```python
from build123d import *

# Parameters (mm, degrees)
SKETCH1_R           = 1.5
BOSS_EXTRUDE1_DEPTH = 5
SKETCH2_W           = 3.5
SKETCH2_H           = 1.5
CUT_EXTRUDE1_DEPTH  = 32.689903755


with BuildPart() as part:
    # Sketch1 → Boss-Extrude1 (new body)
    with BuildSketch(Plane.XY):
        with BuildLine():
            Line((0, 0), (27, 0))
            ThreePointArc((27, 0), (30.5, -3.5), (27, -7))
            Line((27, -7), (0, -7))
            ThreePointArc((0, -7), (-3.5, -3.5), (0, 0))
        make_face()
        with Locations((0, -3.5)):
            Circle(SKETCH1_R, mode=Mode.SUBTRACT)
        with Locations((27, -3.5)):
            Circle(SKETCH1_R, mode=Mode.SUBTRACT)
    extrude(amount=BOSS_EXTRUDE1_DEPTH)

    # Sketch2 → Cut-Extrude1 (cut, through all)
    with BuildSketch(Plane(origin=(0, 0, 0), x_dir=(1, 0, 0), z_dir=(0, 1, 0))):
        Polygon((0, -5), (14.5, -5), (13, -3.5), (0, -3.5), align=None)
        Polygon((15.949747468, -1.5), (27, -1.5), (27, 0), (14.449747468, 0), align=None)
        with Locations((-1.75, -4.25)):
            Rectangle(SKETCH2_W, SKETCH2_H)
        with Locations((28.75, -0.75)):
            Rectangle(SKETCH2_W, SKETCH2_H)
    extrude(amount=-CUT_EXTRUDE1_DEPTH, mode=Mode.SUBTRACT)


solid = part.part
```
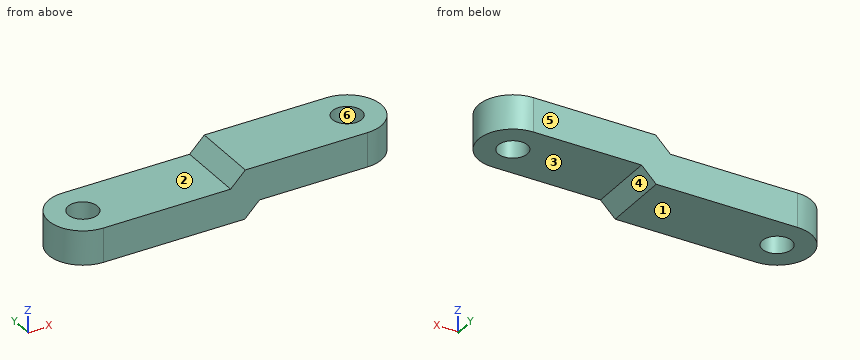
Geometry check sheet. Reference: the model listing, model coordinates, mm. Face numbers are marked on the shaded views. A direction names the side the tool comes from. Give positions to 0.01 mm unless a question says otherwise; leave off trailing zeros. Order: outer loops, then holes, each group sorted by start corner. A loop starts at its lowest first (then second) coordinate and runs counter-clockwise, first axis right, second up. Notation, with made-up numbers: (-20, 47) -> (14, 47) arc R10 ccw to (14, 63) -> close; hole circle Ø6 at (-19, 11.25). An arc over 180 degrees is marked (long way). Write each question's results on one line, items separated by ' | '. Start each with the question number.
(1) Mould release check, pull along Y, two halves, no side actions. Record for the marked faces 4, 5 and 6: pulls with the +Y half, pulls with the -Y half, needs draft (parallel to the pull), parting line crosses it, or undercut.
(2) Gauge pin test, flat ends, axial feed: P1, Ø1, axis at y = -5, z = 4.5, coming from the +X side; P2, Ø3.5, axis at x = 8, y = -2.5, coming from the +Z side; P3, Ø1, axis at y = -6, z = 2.5, coming from the +X side. Record the tip position at first contact, or that the pin passes through.
(3) Access from +Z, -Z, +X, -X, +Y, -Y to the whole of each face (thin tool, end or side, straight path). Record for the marked faces 1, 2 and 3.
(4) Sectioned sample at D-D (y = -6). Enter the section's corners in (x, z), plus the area to 3 significant figures.
(5) Scan lines: line 1 (X direction, y = -3.5, z = 2.3); line 2 (X direction, y = -4.5, z = 2.5); line 3 (Y direction, x = 0, z = 1.85). Record each from-to range of solid material in increasing order.
(6) Sectioned sample at B-B (z = 4.3). Enter the section's corners in (x, y).
(7) Sectioned sample at C-C (x = 4.5). Enter the section's corners in (y, z), plus the area to 3 significant figures.
(8) Sectioned sample at A-A (y = -3.5). Enter the section's corners in (x, z).
Answer below:
1) face 4: needs draft | face 5: pulls with the +Y half | face 6: undercut
2) P1: x = 30.35 | P2: z = 3.5 | P3: x = 29.87
3) face 1: -Z, +X, -X, +Y, -Y | face 2: +Z, -X, +Y, -Y | face 3: -Z, +X, +Y, -Y
4) outline: (-2.45, 0) -> (14.45, 0) -> (15.95, 1.5) -> (29.45, 1.5) -> (29.45, 5) -> (14.5, 5) -> (13, 3.5) -> (-2.45, 3.5) -> close | area: 114 mm2
5) line 1: -3.5 to -1.5, 1.5 to 25.5, 28.5 to 30.5 | line 2: -3.35 to -1.12, 1.12 to 25.88, 28.12 to 30.35 | line 3: -7 to -5, -2 to 0
6) outline: (13.8, -7) -> (27, -7) arc R3.5 ccw to (27, 0) -> (13.8, 0) -> close; hole circle Ø3 at (27, -3.5)
7) outline: (-7, 0) -> (0, 0) -> (0, 3.5) -> (-7, 3.5) -> close | area: 24.5 mm2
8) outline: (-3.5, 0) -> (-1.5, 0) -> (-1.5, 3.5) -> (-3.5, 3.5) -> close; (1.5, 0) -> (14.45, 0) -> (15.95, 1.5) -> (25.5, 1.5) -> (25.5, 5) -> (14.5, 5) -> (13, 3.5) -> (1.5, 3.5) -> close; (28.5, 1.5) -> (30.5, 1.5) -> (30.5, 5) -> (28.5, 5) -> close
